Input: dimensioned drawing with shaded views. Units: mm. Origin: part minimum x, y, z. A direction names the side the tool comes from. Coordinates: 2 decimals unless noted, no trailing zeros. Loops run counter-clockwise (first coordinate to the right, second up) from the corner with the lowest first, then second, coordinate; pieces in that order, holes last.
(1) Section D-D, the plane z = 36. Return loops of the section in (x, y).
(2) Mould query, pull axis Z, two halves, no side actions, for the marked faces 1, 2, 3 and 4. Classes: released by +Z, released by -Z, zero draft, split by the parting line, or undercut.
(3) Section C-C, the plane z = 57. Return loops of the section in (x, y).
(4) Line query: L1, parallel to X at y = 6.5, z = 12; L2, parallel to Z at x = 107, y = 5.75; L3, parallel to X at y = 4.5, z = 9. Output: solid intervals per line, ascending.
(5) Section A-A, the plane y = 3.5. Return loops of the section in (x, z).
(6) Contact query for flat-ended pins moving along their axis: P1, Ø6, axis at x = 77.5, y = 1.5, coming from the +Z side; P2, Ø19, axis at x = 108, z = 60, coming from the -Y side; P3, Ø10, axis at x = 18.5, z = 31.5, coming from the +Y side; P4, Ø0.9, axis at y = 11.5, z = 21.5, coming from the -X side. Output: stop coordinate, or through.
(7) Section B-B, the plane x = 8. Return loops of the section in (y, z), then the cut area to 3 significant figures.
(8) Set-up query: the marked faces 5, 6, 7 and 8. Return all of +Z, -Z, +X, -X, +Y, -Y with unobstructed straight access to the full face (end or side cutting, diameter ignored); none if empty.
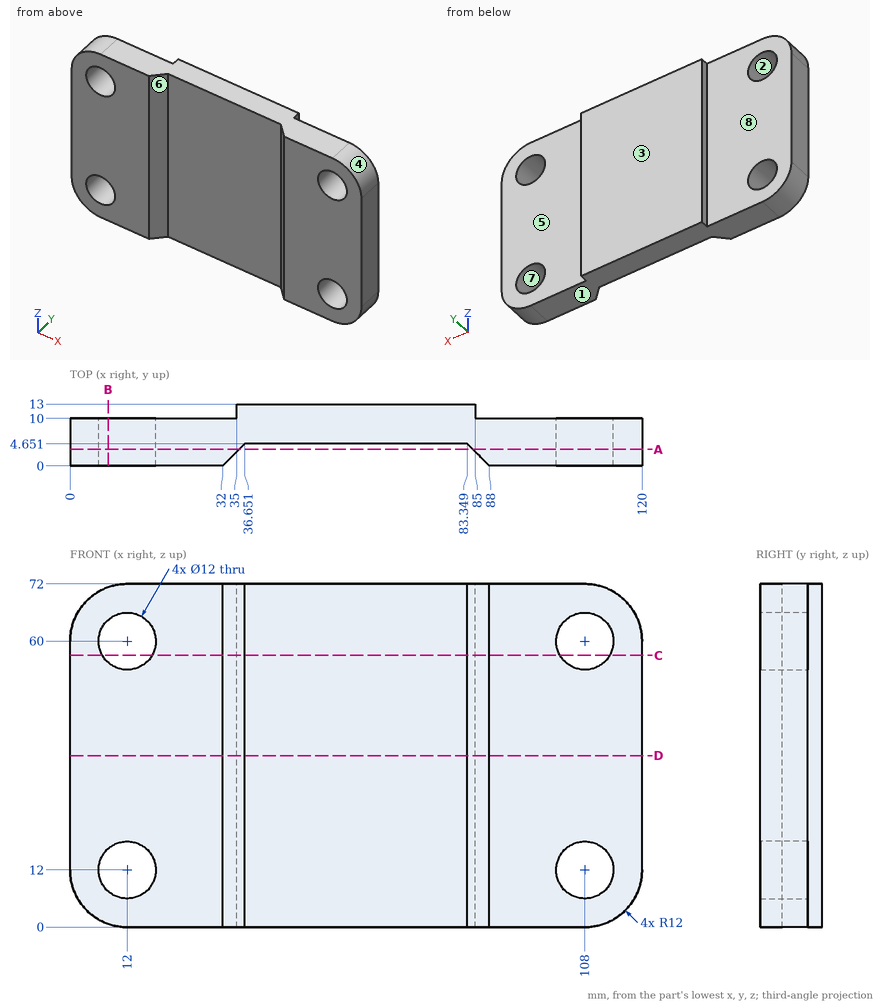
Report:
1. outline: (0, 0) - (32, 0) - (36.65, 4.65) - (83.35, 4.65) - (88, 0) - (120, 0) - (120, 10) - (85, 10) - (85, 13) - (35, 13) - (35, 10) - (0, 10) - close
2. face 1: released by -Z
2. face 2: undercut
2. face 3: zero draft
2. face 4: released by +Z
3. outline: (0, 0) - (6.8, 0) - (6.8, 10) - (0, 10) - close; (17.2, 0) - (32, 0) - (36.65, 4.65) - (83.35, 4.65) - (88, 0) - (102.8, 0) - (102.8, 10) - (85, 10) - (85, 13) - (35, 13) - (35, 10) - (17.2, 10) - close; (113.2, 0) - (120, 0) - (120, 10) - (113.2, 10) - close
4. L1: x = 0 to 6, 18 to 102, 114 to 120
4. L2: z = 0 to 6.08, 17.92 to 54.08, 65.92 to 72
4. L3: x = 0.38 to 6.8, 17.2 to 36.5, 83.5 to 102.8, 113.2 to 119.62
5. outline: (0, 12) arc R12 ccw to (12, 0) - (35.5, 0) - (35.5, 72) - (12, 72) arc R12 ccw to (0, 60) - close; (84.5, 0) - (108, 0) arc R12 ccw to (120, 12) - (120, 60) arc R12 ccw to (108, 72) - (84.5, 72) - close; hole circle Ø12 at (12, 12); hole circle Ø12 at (12, 60); hole circle Ø12 at (108, 12); hole circle Ø12 at (108, 60)
6. P1: passes through
6. P2: stops at y = 0
6. P3: stops at y = 10
6. P4: stops at x = 35
7. outline: (0, 0.69) - (10, 0.69) - (10, 7.53) - (0, 7.53) - close; (0, 16.47) - (10, 16.47) - (10, 55.53) - (0, 55.53) - close; (0, 64.47) - (10, 64.47) - (10, 71.31) - (0, 71.31) - close
7. area: 527 mm2
8. face 5: +Z, -Z, +X, +Y
8. face 6: +Z, -Z, -Y
8. face 7: +Y, -Y
8. face 8: +Z, -Z, -X, +Y
